Design review of the part built by this model. Coordinates are the model's own, in mm. A direction names the side the tool comes from. Give positions to 0.01 mm unless a question says otherwise; leave off trailing zeros. Order: outer loops, then holes, each group sorted by start corner. A loop starts at its lowest first (then second) coordinate and runs counter-clockwise, first axis right, second up. Notation, with made-up numbers: (9, -11.5) -> (31, -11.5) arc R23 ccw to (31, 4.5) -> close; hole circle Ø11 at (63, 68.25). An arc over 180 degrees is marked (long way). Use a Markdown table: item, result. Add a question column.
```python
from build123d import *

# Parameters (mm, degrees)
SKETCH1_W           = 150
SKETCH1_H           = 37.75
BOSS_EXTRUDE1_DEPTH = 18
SKETCH2_W           = 12
SKETCH2_H           = 5.9
CUT_EXTRUDE1_DEPTH  = 150
SKETCH3_W           = 12
SKETCH3_H           = 5.9
CUT_EXTRUDE2_DEPTH  = 150
SKETCH4_W           = 140.2
SKETCH4_H           = 10.2
CUT_EXTRUDE3_DEPTH  = 7.5


with BuildPart() as part:
    # Sketch1 → Boss-Extrude1 (new body)
    with BuildSketch(Plane(origin=(0, 0, 0), x_dir=(1, 0, 0), z_dir=(0, 1, 0))):
        Rectangle(SKETCH1_W, SKETCH1_H)
    extrude(amount=BOSS_EXTRUDE1_DEPTH)

    # Sketch2 → Cut-Extrude1 (cut)
    with BuildSketch(Plane(origin=(75, 0, 0), x_dir=(0, 0, -1), z_dir=(1, 0, 0))):
        with Locations((-12.875, 15.05)):
            Rectangle(SKETCH2_W, SKETCH2_H)
    extrude(amount=-CUT_EXTRUDE1_DEPTH, mode=Mode.SUBTRACT)

    # Sketch3 → Cut-Extrude2 (cut)
    with BuildSketch(Plane(origin=(75, 0, 0), x_dir=(0, 0, -1), z_dir=(1, 0, 0))):
        with Locations((12.875, 15.05)):
            Rectangle(SKETCH3_W, SKETCH3_H)
    extrude(amount=-CUT_EXTRUDE2_DEPTH, mode=Mode.SUBTRACT)

    # Sketch4 → Cut-Extrude3 (cut)
    with BuildSketch(Plane.XZ):
        Rectangle(SKETCH4_W, SKETCH4_H)
    extrude(amount=-CUT_EXTRUDE3_DEPTH, mode=Mode.SUBTRACT)


solid = part.part
```
1) Add section D-D (y = 15.75). Give the boundary of the cut face in (x, z) (3 decimals).
2) Add section B-B (z = -2). Give the boundary of the cut face in (x, y), then the cut area to 3 significant figures.
3) Add section A-A (y = 2.25). Give the boundary of the cut face in (x, z) (3 decimals), then the cut area to 3 significant figures.
4) The part is to be moulded in two halves that separate along Z. For faces 1 (the flat face through (-1, 4, -5.1)), 2 (the flat face through (-1, 7.5, 0)), 3 (the flat face through (75, 7, 0)), 4 (the flat face through (-1, 6, -18.875)), say which applies: +Z half, -Z half, draft (parallel to the pull), parting line (faces both ways), or undercut.
5) Add section C-C (x = 2.5). Give the boundary of the cut face in (y, z) (3 decimals), then the cut area to 3 significant figures.
6) For L1, parallel to Z at x = -31, y = 2.5 (3 decimals); L2, parallel to Y at x = 23, z = 1.5; L3, parallel to Z at x = -7.5, y = 13 (3 decimals), list the stretches that pass through material, from the lowest coordinate up. Write a range as [from, to].
7) Machinability: for faces 5 (the flat face through (1, 12.1, -13)), 6 (the flat face through (-1, 6, 18.875)), 7 (the flat face through (-1, 4, 5.1)), 8 (the flat face through (1, 12.1, 13)), which of the approach directions +Z, -Z, +X, -X, +Y, -Y give a long, thin tool a straight path to every point of the face, cutting with its end or side? Answer none if there is none.
8) Insertion check: pin 1 (3 mm diameter, centred on x = 11.5, z = -1, fed in from -Y); pin 2 (3 mm diameter, centred on x = 34.5, y = 16.5, fed in from +Z) (3 decimals); pin 3 (1.8 mm diameter, centred on x = 30, y = 15, fed in from -Z) (3 decimals). Each pin has a flat end and moves straight along its axis. Give the tip position at first contact, or say it passes through.
Worked answers:
| question | item | result |
|---|---|---|
| 1 | outline | (-75, -6.875) -> (75, -6.875) -> (75, 6.875) -> (-75, 6.875) -> close |
| 2 | outline | (-75, 0) -> (-70.1, 0) -> (-70.1, 7.5) -> (70.1, 7.5) -> (70.1, 0) -> (75, 0) -> (75, 18) -> (-75, 18) -> close |
| 2 | area | 1,650 mm^2 |
| 3 | outline | (-75, -18.875) -> (75, -18.875) -> (75, 18.875) -> (-75, 18.875) -> close; hole (-70.1, -5.1) -> (70.1, -5.1) -> (70.1, 5.1) -> (-70.1, 5.1) -> close |
| 3 | area | 4,230 mm^2 |
| 4 | face 1 | undercut |
| 4 | face 2 | undercut |
| 4 | face 3 | draft |
| 4 | face 4 | -Z half |
| 5 | outline | (0, -18.875) -> (12.1, -18.875) -> (12.1, -6.875) -> (18, -6.875) -> (18, 6.875) -> (12.1, 6.875) -> (12.1, 18.875) -> (0, 18.875) -> (0, 5.1) -> (7.5, 5.1) -> (7.5, -5.1) -> (0, -5.1) -> close |
| 5 | area | 461 mm^2 |
| 6 | L1 | [-18.875, -5.1], [5.1, 18.875] |
| 6 | L2 | [7.5, 18] |
| 6 | L3 | [-6.875, 6.875] |
| 7 | face 5 | -Z, +X, -X, +Y |
| 7 | face 6 | +Z, +X, -X, +Y, -Y |
| 7 | face 7 | -Y |
| 7 | face 8 | +Z, +X, -X, +Y |
| 8 | pin 1 | y = 7.5 |
| 8 | pin 2 | z = 6.875 |
| 8 | pin 3 | z = -6.875 |
